Verification items for the finished model (mm, model axes). Face numbers are marked on the shaded views. A direction names the side the tool comes from. Round coordinates to 2 decimals unless told otherwise and drop trailing zeros. Order: outer loops, then holes, each group sorted by start corner. A loop starts at its lowest first (then second) coordinate and runs counter-clockwise, first axis right, second up. Notation, with made-up numbers: M 0.5,-25 L 38.5,-25 A15 ccw 38.5,-4 Z; hole C 25.5,-18 d1. An arc over 180 degrees is marked long. Use CSV: the item, a comma, the result in double quotes. Start each with the question number.
Q1. Mould release check, pull along Z, two halves, no side actions. Record for the marked faces 5 and 6: +Z half, -Z half, draft (parallel to the pull), parting line (faces both ways), or undercut.
Q2. Sectioned sample at C-C (z = 14). Enter the section's corners in (x, y), and give its area (3 significant figures).
Q3. Sectioned sample at A-A (y = -10). Enter the section's corners in (x, z), and give its area (3 significant figures).
Q4. Scan lines: line 1 (Y direction, x = 11.5, z = 10.25); line 2 (X direction, y = 37, z = 17.5); line 3 (Y direction, x = -14.5, z = 12.5). Record each from-to range of solid material in increasing order.
Q5. Gauge pin test, flat ends, axial feed: pin 1 Ø0.9 at (y, z) = (-23, 2) entering from +X; pin 2 Ø3 at (x, y) = (0.5, -5.5) entering from -Z; pin 3 Ø9.5 at (y, z) = (23, 19) entering from +X; pin 4 Ø5 at (y, z) = (8.5, 12.5) entering from +X. Record the tip position at first contact, or that the pin passes through.
Q6. Set-up check for the marked faces 1, 2, 3 and 4: record each of +Z, -Z, +X, -X, +Y, -Y from which the full face is reachable in a straight line by a thin tool's end or side.
Q7. Sectioned sample at B-B (x = 8.5). State how many separate pieces and enclosed holes the cut face has, and give its area (3 significant figures).
```python
from build123d import *

# Parameters (mm, degrees)
F1_DEPTH = 3
F2_DEPTH = 25
F3_R     = 3


with BuildPart() as f1:
    # F0 (on Top) → F1 (new body)
    with BuildSketch(Plane.XY):
        Polygon((-21, -35), (5, -35), (5, -5), (27, -5), (27, 21), (5, 21), (5, 24), (34, 24), (34, 50), (-21, 50), align=None)
        Polygon((-16.7, 45.7), (29.7, 45.7), (29.7, 28.3), (0.7, 28.3), (0.7, 16.7), (22.7, 16.7), (22.7, -0.7), (0.7, -0.7), (0.7, -30.7), (-16.7, -30.7), align=None, mode=Mode.SUBTRACT)
        Polygon((29.7, 28.3), (29.7, 45.7), (-16.7, 45.7), (-16.7, -30.7), (0.7, -30.7), (0.7, -0.7), (22.7, -0.7), (22.7, 16.7), (0.7, 16.7), (0.7, 28.3), align=None)
        Polygon((22, 0), (0, 0), (0, -30), (-16, -30), (-16, 45), (29, 45), (29, 29), (0, 29), (0, 16), (22, 16), align=None, mode=Mode.SUBTRACT)
        Polygon((0, -30), (0, 0), (22, 0), (22, 16), (0, 16), (0, 29), (29, 29), (29, 45), (-16, 45), (-16, -30), align=None)
        Polygon((21, 1), (-1, 1), (-1, -29), (-15, -29), (-15, 44), (28, 44), (28, 30), (-1, 30), (-1, 15), (21, 15), align=None, mode=Mode.SUBTRACT)
    extrude(amount=F1_DEPTH)

    # F0 (on Top) → F2 (join)
    with BuildSketch(Plane.XY):
        Polygon((29.7, 28.3), (29.7, 45.7), (-16.7, 45.7), (-16.7, -30.7), (0.7, -30.7), (0.7, -0.7), (22.7, -0.7), (22.7, 16.7), (0.7, 16.7), (0.7, 28.3), align=None)
        Polygon((22, 0), (0, 0), (0, -30), (-16, -30), (-16, 45), (29, 45), (29, 29), (0, 29), (0, 16), (22, 16), align=None, mode=Mode.SUBTRACT)
    extrude(amount=F2_DEPTH)

    # F3
    f3_edges = [f1.edges().sort_by_distance(p)[0] for p in [
        (27, 21, 1.5),
        (-1, 15, 1.5),
        (27, -5, 1.5),
        (5, -35, 1.5),
        (-21, -35, 1.5),
        (-21, 50, 1.5),
        (34, 24, 1.5),
        (34, 50, 1.5),
        (-1, 30, 1.5),
        (-1, 1, 1.5),
        (-1, -29, 1.5),
        (-15, -29, 1.5),
        (21, 1, 1.5),
        (21, 15, 1.5),
        (28, 30, 1.5),
        (28, 44, 1.5),
        (-15, 44, 1.5),
    ]]
    fillet(f3_edges, radius=F3_R)


solid = f1.part
```
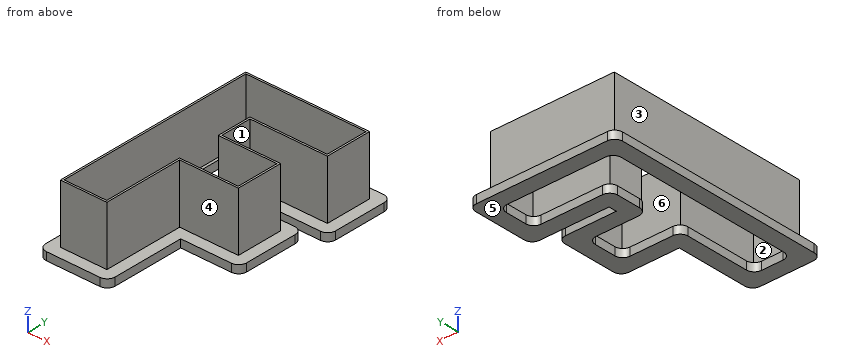
Verdict:
1,face 5,"-Z half"
1,face 6,"draft"
2,outline,"M -16.7,-30.7 L 0.7,-30.7 L 0.7,-0.7 L 22.7,-0.7 L 22.7,16.7 L 0.7,16.7 L 0.7,28.3 L 29.7,28.3 L 29.7,45.7 L -16.7,45.7 Z; hole M -16,-30 L 0,-30 L 0,0 L 22,0 L 22,16 L 0,16 L 0,29 L 29,29 L 29,45 L -16,45 Z"
2,area,"201 mm²"
3,outline,"M -21,0 L -15,0 L -15,3 L -16,3 L -16,25 L -16.7,25 L -16.7,3 L -21,3 Z; M -1,0 L 5,0 L 5,3 L 0.7,3 L 0.7,25 L 0,25 L 0,3 L -1,3 Z"
3,area,"66.8 mm²"
4,line 1,"y = -0.7 to 0, 16 to 16.7, 28.3 to 29, 45 to 45.7"
4,line 2,"x = -16.7 to -16, 29 to 29.7"
4,line 3,"y = -30.7 to -30, 45 to 45.7"
5,pin 1,"stops at x = 5"
5,pin 2,"stops at z = 0"
5,pin 3,"stops at x = 0.7"
5,pin 4,"stops at x = 22.7"
6,face 1,"+Z, +X"
6,face 2,"+Z"
6,face 3,"+Z, -X, +Y, -Y"
6,face 4,"+Z, +X, -Y"
7,separate pieces,"4"
7,enclosed holes,"0"
7,area,"134 mm²"
